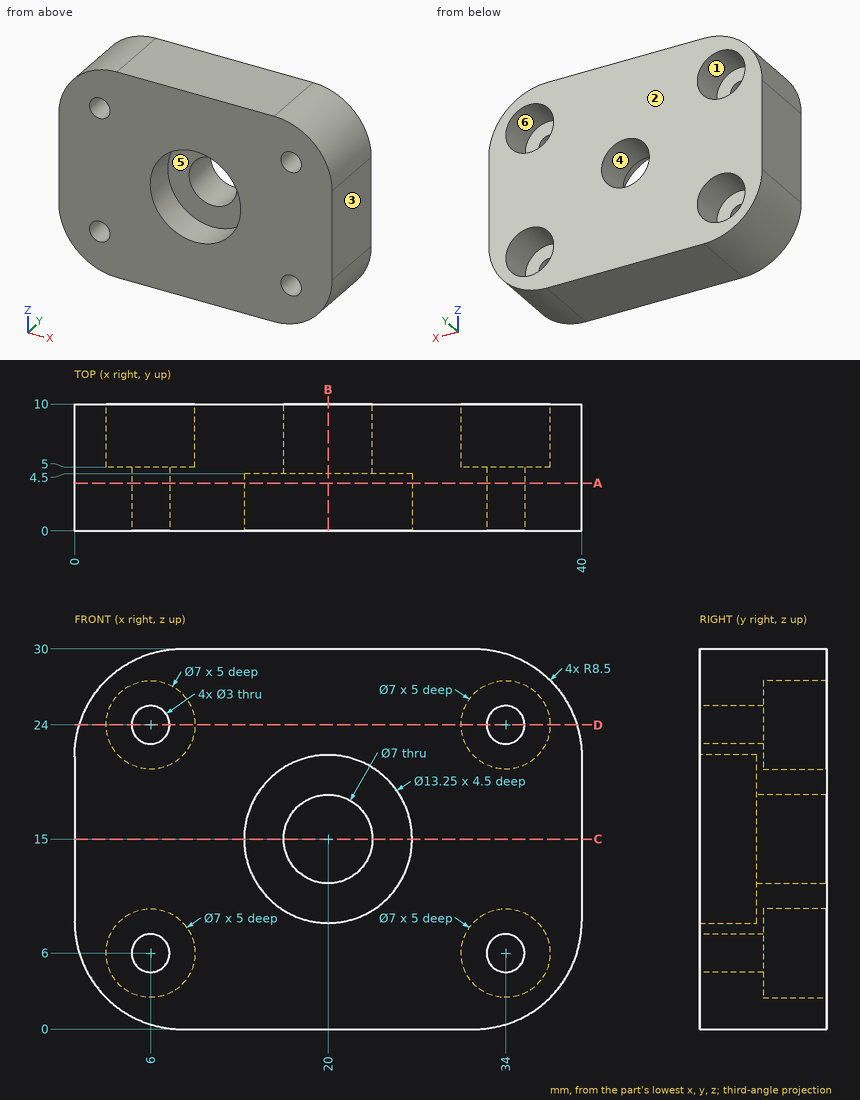
Here's the drawing with two shaded views (mm, measured from the low corner). I have some questions. A direction names the side the tool comes from. Coordinates: 2 decimals unless noted, no trailing zeros. Order: outer loops, then holes, each group sorted by start corner. A loop starts at its lowest first (then second) coordinate and runs counter-clockwise, first axis right, second up. Notation, with made-up numbers: (3, 51) - (13, 51) arc R12 cw to (13, 66) - close; hole circle Ø2 at (4, 74.25). An arc over 180 degrees is marked (long way). Answer in a Markdown table with one row per item. Add a question column.
(1) If we section it at A-A, the plane y = 3.75: Please give me the cut outline in (x, z) (3 decimals).
(2) Will these pins go through, and if not, where does the flat tip stop? pin 1 (9 mm diameter, centred on x = 20, z = 15, fed in from -Y); pin 2 (1.5 mm diameter, centred on y = 3, z = 24.5, fed in from -X); pin 3 (2 mm diameter, centred on x = 7, z = 23.5, fed in from +Y).
(3) If we section it at D-D, the plane z = 24: Please give me the cut outline in (x, y).
(4) I need wall thicknesses on L1, parallel to Z at x = 6, y = 1.75; L2, parallel to X at y = 9, z = 26; L3, parallel to X at y = 8.75, z = 5. Which ranges of each line are inside material? Lowest first, please.
(5) If we mould it in two halves opening along X, with no side actions, what happens to the marked faces 1, 2 and 3? For each: released by +X, released by -X, zero draft, split by the parting line, or undercut.
(6) If we section it at B-B, the plane x = 20: Please give me the cut outline in (y, z) (3 decimals).
(7) If we section it at C-C, the plane z = 15: Please give me the cut outline in (x, y) (3 decimals).
(8) On a 3-axis mill with a long thin cutter (end or side, diameter ignored), from which of +Z, -Z, +X, -X, +Y, -Y can I reach the whole of each face in a straight line? I mean the marked faces 4, 5 and 6. Say none if no direction works.
Results are:
| question | item | result |
|---|---|---|
| 1 | outline | (0, 8.5) arc R8.5 ccw to (8.5, 0) - (31.5, 0) arc R8.5 ccw to (40, 8.5) - (40, 21.5) arc R8.5 ccw to (31.5, 30) - (8.5, 30) arc R8.5 ccw to (0, 21.5) - close; hole circle Ø3 at (6, 6); hole circle Ø3 at (6, 24); hole circle Ø13.25 at (20, 15); hole circle Ø3 at (34, 6); hole circle Ø3 at (34, 24) |
| 2 | pin 1 | stops at y = 4.5 |
| 2 | pin 2 | stops at x = 0.3 |
| 2 | pin 3 | stops at y = 5 |
| 3 | outline | (0.38, 0) - (4.5, 0) - (4.5, 5) - (2.5, 5) - (2.5, 10) - (0.38, 10) - close; (7.5, 0) - (32.5, 0) - (32.5, 5) - (30.5, 5) - (30.5, 10) - (9.5, 10) - (9.5, 5) - (7.5, 5) - close; (35.5, 0) - (39.62, 0) - (39.62, 10) - (37.5, 10) - (37.5, 5) - (35.5, 5) - close |
| 4 | L1 | z = 0.38 to 4.5, 7.5 to 22.5, 25.5 to 29.62 |
| 4 | L2 | x = 1.29 to 3.13, 8.87 to 31.13, 36.87 to 38.71 |
| 4 | L3 | x = 0.75 to 2.65, 9.35 to 30.65, 37.35 to 39.25 |
| 5 | face 1 | undercut |
| 5 | face 2 | zero draft |
| 5 | face 3 | released by +X |
| 6 | outline | (0, 0) - (10, 0) - (10, 11.5) - (4.5, 11.5) - (4.5, 8.375) - (0, 8.375) - close; (0, 21.625) - (4.5, 21.625) - (4.5, 18.5) - (10, 18.5) - (10, 30) - (0, 30) - close |
| 7 | outline | (0, 0) - (13.375, 0) - (13.375, 4.5) - (16.5, 4.5) - (16.5, 10) - (0, 10) - close; (23.5, 4.5) - (26.625, 4.5) - (26.625, 0) - (40, 0) - (40, 10) - (23.5, 10) - close |
| 8 | face 4 | +Y, -Y |
| 8 | face 5 | -Y |
| 8 | face 6 | +Y |
